Could you check a few things on this model? Use its own coordinates, in mm. A direction names the side the tool comes from. Coordinates: 2 decimals unless noted, no trailing zeros. Order: outer loops, then holes, each group sorted by start corner. A loop starts at its lowest first (then second) coordinate and runs counter-clockwise, first axis right, second up. Notation, with made-up numbers: (-35.75, 51.25) - (16.25, 51.25) arc R29 cw to (16.25, 85.25) - close; hole circle Ø10 at (6, -20). An arc over 180 degrees is marked (long way). Answer as a JSON object with one key per item and string values. Group by question number.
(1) Imagine slicing it at A-A, the plane z = 0. Write out the boundary of the cut face in (x, y) (3 decimals), and give its area (3 significant figures).
(2) Please list where these lines run through material, in increasing order: probe 1 along X at (y, z) = (0.85, 0.75); probe 2 along X at (y, z) = (0.3, -8); probe 3 along X at (y, z) = (0.2, -0.5).
(3) Imagine slicing it at D-D, the plane x = 6.35. Write out the boundary of the cut face in (y, z), and give its area (3 significant figures).
(4) Which directions (+Z, -Z, +X, -X, +Y, -Y) give clear straight access to the entire face, cutting with the end or side of a thin tool? Please do faces 4 (the cylindrical face through (-9.94, 2.03, 7.19)), 5 (the cylindrical face through (-8.84, 0.44, -5.88)), 6 (the flat face through (12, 1, -8.954)), 7 (the flat face through (-10.033, 1, 0)).
(5) Will these pins go through, and if not, where does the flat tip stop? P1, Ø3, axis at x = 17.83, z = -5.68, coming from the +Y side; P2, Ø1, axis at x = -10, z = -5, coming from the -Y side; P3, Ø9, axis at x = 0.5, z = -1.5, coming from the +Y side.
(6) We'd pull the mould along Z, two halves only. Please class faces 1 (the flat face through (0, 1, 8.954)), 2 (the cylindrical face through (6.3, 0.81, -6.54)), 3 (the flat face through (-20.447, 1, 0)): pulls with the +Z half, pulls with the -Z half, needs draft (parallel to the pull), parting line crosses it, or undercut.
(7) Imagine slicing it at C-C, the plane z = 7.75. Write out the boundary of the cut face in (x, y), and give its area (3 significant figures).
from build123d import *

# Parameters (mm, degrees)
SKETCH1_R           = 1.3335
SKETCH1_R_2         = 1.5875
BOSS_EXTRUDE1_DEPTH = 1.651
CHAMFER1_SIZE       = 2.54
SKETCH1_2_R         = 1.5875
BOSS_EXTRUDE2_DEPTH = 2.413
SKETCH1_3_R         = 1.5875
CUT_EXTRUDE1_DEPTH  = 0.889
CUT_EXTRUDE3_DEPTH  = 23.382376376
SKETCH4_R           = 2.413
BOSS_EXTRUDE3_DEPTH = 0.381
CUT_EXTRUDE4_START  = -1.651
SKETCH4_2_R         = 2.413
CUT_EXTRUDE4_DEPTH  = 0.635


with BuildPart() as part:
    # Sketch1 → Boss-Extrude1 (new body)
    with BuildSketch(Plane(origin=(0, 0, 0), x_dir=(1, 0, 0), z_dir=(0, 1, 0))):
        with BuildLine():
            Line((-5.567119422, 8.9535), (5.567119422, 8.9535))
            ThreePointArc((5.567119422, 8.9535), (6.35, 6.5405), (7.132880578, 8.9535))
            Line((7.132880578, 8.9535), (20.447, 8.9535))
            Line((20.447, 8.9535), (20.447, -8.9535))
            Line((20.447, -8.9535), (7.132880578, -8.9535))
            ThreePointArc((7.132880578, -8.9535), (6.35, -6.5405), (5.567119422, -8.9535))
            Line((5.567119422, -8.9535), (-5.567119422, -8.9535))
            ThreePointArc((-5.567119422, -8.9535), (-6.35, -6.5405), (-7.132880578, -8.9535))
            Line((-7.132880578, -8.9535), (-20.447, -8.9535))
            Line((-20.447, -8.9535), (-20.447, 8.9535))
            Line((-20.447, 8.9535), (-7.132880578, 8.9535))
            ThreePointArc((-7.132880578, 8.9535), (-6.35, 6.5405), (-5.567119422, 8.9535))
        make_face()
        with Locations(Location((-17.8308, 5.6769, 0), (0, 0, 90))):
            Circle(SKETCH1_R, mode=Mode.SUBTRACT)
        with Locations(Location((17.8308, 5.6769, 0), (0, 0, 90))):
            Circle(SKETCH1_R, mode=Mode.SUBTRACT)
        with Locations(Location((17.8308, -5.6769, 0), (0, 0, 90))):
            Circle(SKETCH1_R, mode=Mode.SUBTRACT)
        with Locations(Location((-17.8308, -5.6769, 0), (0, 0, 90))):
            Circle(SKETCH1_R, mode=Mode.SUBTRACT)
        with Locations(Location((-10.414, 5.6769, 0), (0, 0, 90))):
            Circle(SKETCH1_R_2, mode=Mode.SUBTRACT)
        with Locations(Location((10.414, 5.6769, 0), (0, 0, 90))):
            Circle(SKETCH1_R_2, mode=Mode.SUBTRACT)
        with Locations(Location((10.414, -5.6769, 0), (0, 0, 90))):
            Circle(SKETCH1_R_2, mode=Mode.SUBTRACT)
        with Locations(Location((-10.414, -5.6769, 0), (0, 0, 90))):
            Circle(SKETCH1_R_2, mode=Mode.SUBTRACT)
    extrude(amount=BOSS_EXTRUDE1_DEPTH)

    # Chamfer1
    chamfer1_edges = [part.edges().sort_by_distance(p)[0] for p in [
        (20.447, 0.8255, -8.9535),
        (20.447, 0.8255, 8.9535),
        (-20.447, 0.8255, 8.9535),
        (-20.447, 0.8255, -8.9535),
    ]]
    chamfer(chamfer1_edges, length=CHAMFER1_SIZE)

    # Sketch1<2> → Boss-Extrude2 (add)
    with BuildSketch(Plane(origin=(0, 0, 0), x_dir=(1, 0, 0), z_dir=(0, 1, 0))):
        with Locations(Location((-10.414, 5.6769, 0), (0, 0, 270))):
            Circle(SKETCH1_2_R)
        with Locations(Location((10.414, 5.6769, 0), (0, 0, 270))):
            Circle(SKETCH1_2_R)
        with Locations(Location((10.414, -5.6769, 0), (0, 0, 270))):
            Circle(SKETCH1_2_R)
        with Locations(Location((-10.414, -5.6769, 0), (0, 0, 270))):
            Circle(SKETCH1_2_R)
    extrude(amount=BOSS_EXTRUDE2_DEPTH)

    # Sketch1<3> → Cut-Extrude1 (cut)
    with BuildSketch(Plane(origin=(0, 0, 0), x_dir=(1, 0, 0), z_dir=(0, 1, 0))):
        with Locations(Location((-10.414, 5.6769, 0), (0, 0, 270))):
            Circle(SKETCH1_3_R)
        with Locations(Location((10.414, 5.6769, 0), (0, 0, 270))):
            Circle(SKETCH1_3_R)
        with Locations(Location((10.414, -5.6769, 0), (0, 0, 270))):
            Circle(SKETCH1_3_R)
        with Locations(Location((-10.414, -5.6769, 0), (0, 0, 270))):
            Circle(SKETCH1_3_R)
    extrude(amount=CUT_EXTRUDE1_DEPTH, mode=Mode.SUBTRACT)

    # Sketch3 → Cut-Extrude3 (cut, through all)
    with BuildSketch(Plane(origin=(0, 1.651, 0), x_dir=(1, 0, 0), z_dir=(0, 1, 0))):
        Polygon((-10.033, 1.630758795), (-12.339241205, 3.937), (-15.600758795, 3.937), (-17.907, 1.630758795), (-17.907, -1.630758795), (-15.600758795, -3.937), (-12.339241205, -3.937), (-10.033, -1.630758795), align=None)
        Polygon((17.907, 1.630758795), (15.600758795, 3.937), (12.339241205, 3.937), (10.033, 1.630758795), (10.033, -1.630758795), (12.339241205, -3.937), (15.600758795, -3.937), (17.907, -1.630758795), align=None)
    extrude(amount=-CUT_EXTRUDE3_DEPTH, mode=Mode.SUBTRACT)

    # Sketch4 → Boss-Extrude3 (add)
    with BuildSketch(Plane(origin=(0, 1.651, 0), x_dir=(1, 0, 0), z_dir=(0, 1, 0))):
        with Locations(Location((0, 0, 0), (0, 0, 90))):
            Circle(SKETCH4_R)
    extrude(amount=BOSS_EXTRUDE3_DEPTH)

    # Sketch4<2> → Cut-Extrude4 (cut)
    with BuildSketch(Plane(origin=(0, 1.651, 0), x_dir=(1, 0, 0), z_dir=(0, 1, 0)).offset(CUT_EXTRUDE4_START)):
        with Locations(Location((0, 0, 0), (0, 0, 90))):
            Circle(SKETCH4_2_R)
    extrude(amount=CUT_EXTRUDE4_DEPTH, mode=Mode.SUBTRACT)


solid = part.part
Result set:
{
 "1": {"outline": "(-20.447, 0) - (-17.907, 0) - (-17.907, 1.651) - (-20.447, 1.651) - close; (-10.033, 0) - (-2.413, 0) - (-2.413, 0.635) - (2.413, 0.635) - (2.413, 0) - (10.033, 0) - (10.033, 1.651) - (2.413, 1.651) - (2.413, 2.032) - (-2.413, 2.032) - (-2.413, 1.651) - (-10.033, 1.651) - close; (17.907, 0) - (20.447, 0) - (20.447, 1.651) - (17.907, 1.651) - close", "area": "40.3 mm^2"},
 "2": {"probe 1": "x = -20.45 to -17.91, -10.03 to 10.03, 17.91 to 20.45", "probe 2": "x = -18.86 to -7.68, -5.02 to 5.02, 7.68 to 18.86", "probe 3": "x = -20.45 to -17.91, -10.03 to -2.36, 2.36 to 10.03, 17.91 to 20.45"},
 "3": {"outline": "(0, -6.54) - (1.65, -6.54) - (1.65, 6.54) - (0, 6.54) - close", "area": "21.6 mm^2"},
 "4": {"face 4": "+Y", "face 5": "-Y", "face 6": "-Z, +X, -X, +Y, -Y", "face 7": "+Y, -Y"},
 "5": {"P1": "stops at y = 1.65", "P2": "stops at y = 0.89", "P3": "stops at y = 2.03"},
 "6": {"face 1": "pulls with the +Z half", "face 2": "undercut", "face 3": "needs draft"},
 "7": {"outline": "(-19.11, 0) - (-7.68, 0) - (-7.68, 1.65) - (-19.11, 1.65) - close; (-5.02, 0) - (5.02, 0) - (5.02, 1.65) - (-5.02, 1.65) - close; (7.68, 0) - (19.11, 0) - (19.11, 1.65) - (7.68, 1.65) - close", "area": "54.3 mm^2"}
}
